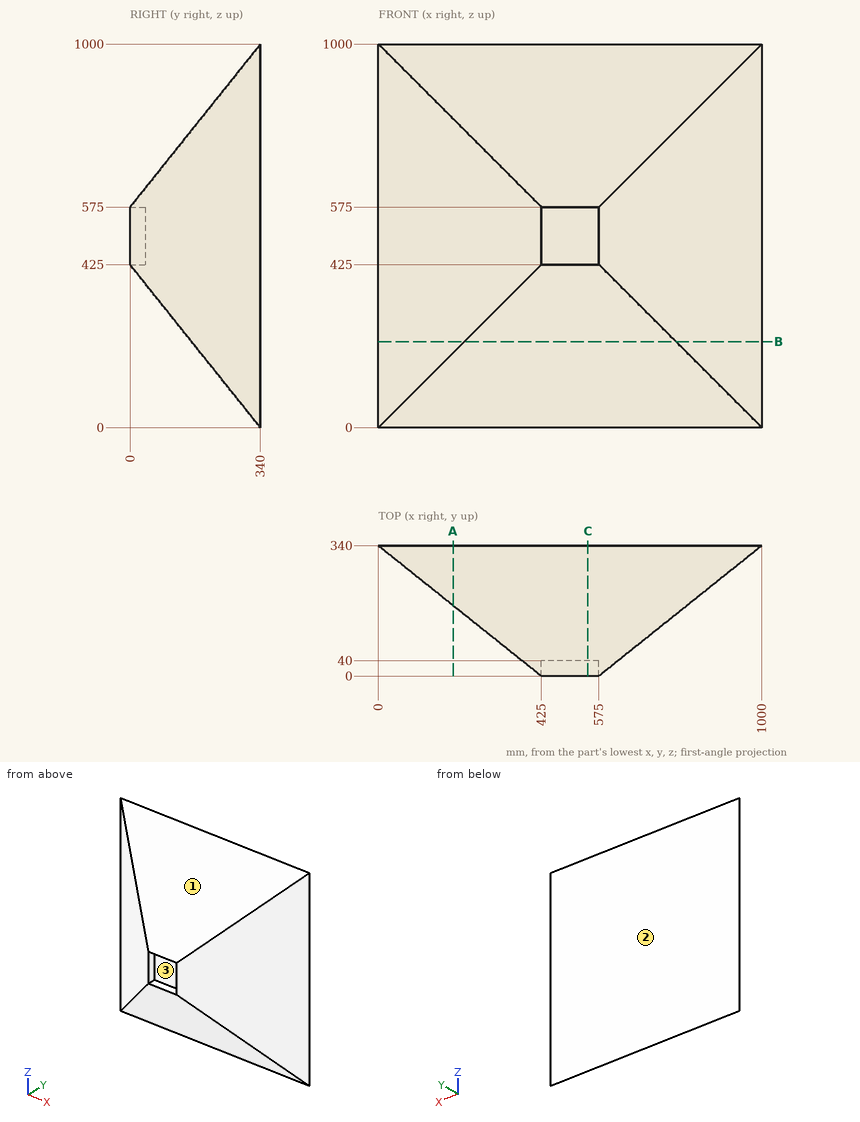
Input: dimensioned drawing with shaded views. Units: mm. Origin: part minimum x, y, z. Round coordinates to 2 decimals unless told otherwise and drop trailing zeros. Order: outer loops, then holes, each group sorted by start corner. A loop starts at its lowest first (then second) coordinate and runs counter-clockwise, first axis right, second up. Notation, with made-up numbers: (-30.5, -33.5) -> (12.5, -33.5) arc R28 cw to (12.5, -11.5) -> close; hole circle Ø11 at (67.25, 36). An arc over 180 degrees is marked (long way). Put each result on its own line as item: value. Start each with the question number.
Q1. Line query: probe 1 along X at (y, z) = (56.5, 620) (3 decimals); probe 2 along X at (y, z) = (238.5, 268.5) (3 decimals); probe 3 along Y at (x, z) = (518, 91). Output: solid intervals per line, ascending.
Q2. Section B-B on z = 224. Return the cut outline in (x, y), and give its area (3 significant figures).
Q3. Pull-direction query (Z, two-part tool) for the marked faces 1, 2 and 3; classes: +Z half, -Z half, draft (parallel to the pull), parting line (faces both ways), or undercut.
Q4. Section C-C on x = 546. Return the cut outline in (y, z), and give its area (4 significant figures).
Q5. Section A-A on x = 195. Return the cut outline in (y, z).
Q6. First-contact query: pin 1 (12 mm diameter, centred on y = 279.5, z = 482.5, fed in from -X) (3 decimals); pin 2 (2 mm diameter, centred on x = 748.5, y = 258.5, fed in from +Z) (3 decimals); pin 3 (12 mm diameter, centred on y = 17.5, z = 520.5, fed in from -X) (3 decimals). Flat tips, straight axial feed; report the tip coordinate or a pass-through.
Ans:
1. probe 1: x = 354.375 to 645.625
1. probe 2: x = 126.875 to 873.125
1. probe 3: y = 267.2 to 340
2. outline: (0, 340) -> (224, 160.8) -> (776, 160.8) -> (1000, 340) -> close
2. area: 139,000 mm2
3. face 1: +Z half
3. face 2: draft
3. face 3: undercut
4. outline: (0, 425) -> (340, 0) -> (340, 1000) -> (0, 575) -> (40, 575) -> (40, 425) -> close
4. area: 189,500 mm2
5. outline: (184, 195) -> (340, 0) -> (340, 1000) -> (184, 805) -> close
6. pin 1: stops at x = 68.125
6. pin 2: stops at z = 899.375
6. pin 3: stops at x = 395.625
